Input: part model. Units: mm. Frame: model coordinates. Face numbers are marked on the shaded views. A direction names the side the tool comes from. Coordinates: 2 decimals unless noted, no trailing zeros. Order: outer loops, then holes, each group sorted by start corner. A loop starts at its lowest first (then second) coordinate and runs counter-clockwise, first axis right, second up. Notation, with made-up numbers: (85.5, -24) -> (105.5, -24) arc R25 ccw to (105.5, 1) -> close; hole circle Ø5 at (72, -36.75). An arc over 180 degrees is marked (long way). Use CSV: the item, a comma, the result in double quotes. Start each with the question number.
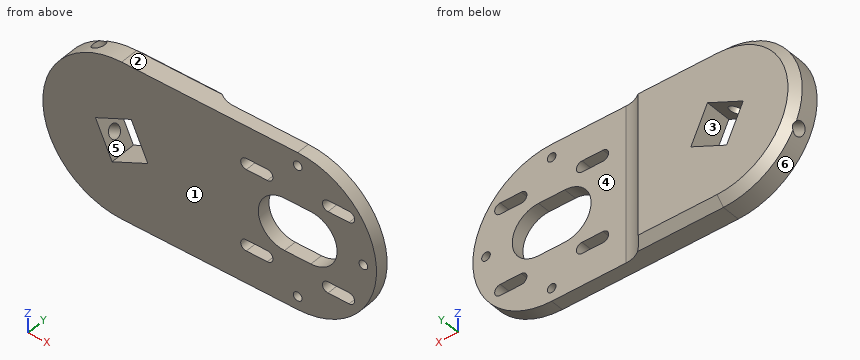
```python
from build123d import *

# Parameters (mm, degrees)
BOSS_EXTRUDE1_DEPTH = 5
CUT_EXTRUDE1_DEPTH  = 71.407741052
BOSS_EXTRUDE2_DEPTH = 5
FILLET1_R           = 10
CUT_EXTRUDE2_DEPTH  = 71.938353519
M4_TAPPED_HOLE1_D   = 3.3
SKETCH13_W          = 2.5
SKETCH13_H          = 32.367781463
SKETCH14_W          = 2.5
SKETCH14_H          = 32.367781463
CHAMFER1_SIZE       = 3


with BuildPart() as part:
    # Sketch1 → Boss-Extrude1 (new body)
    with BuildSketch(Plane(origin=(0, 0, 0), x_dir=(1, 0, 0), z_dir=(0, 1, 0))):
        with BuildLine():
            Line((-33.5, 30), (33.5, 30))
            ThreePointArc((33.5, 30), (63.5, 0), (33.5, -30))
            Line((33.5, -30), (-33.5, -30))
            ThreePointArc((-33.5, -30), (-63.5, 0), (-33.5, 30))
        make_face()
        with BuildLine():
            Line((28.5, 10), (38.5, 10))
            ThreePointArc((38.5, 10), (48.5, 0), (38.5, -10))
            Line((38.5, -10), (28.5, -10))
            ThreePointArc((28.5, -10), (18.5, 0), (28.5, 10))
        make_face(mode=Mode.SUBTRACT)
    extrude(amount=BOSS_EXTRUDE1_DEPTH)

    # Sketch2 → Cut-Extrude1 (cut, through all)
    with BuildSketch(Plane(origin=(0, 5, 0), x_dir=(1, 0, 0), z_dir=(0, 1, 0))):
        with BuildLine():
            Line((13.943650814, 17.686349186), (21.943650814, 17.686349186))
            ThreePointArc((21.943650814, 17.686349186), (24.073650814, 15.556349186), (21.943650814, 13.426349186))
            Line((21.943650814, 13.426349186), (13.943650814, 13.426349186))
            ThreePointArc((13.943650814, 13.426349186), (11.813650814, 15.556349186), (13.943650814, 17.686349186))
        make_face()
        with BuildLine():
            Line((53.056349186, 17.686349186), (45.056349186, 17.686349186))
            ThreePointArc((45.056349186, 17.686349186), (42.926349186, 15.556349186), (45.056349186, 13.426349186))
            Line((45.056349186, 13.426349186), (53.056349186, 13.426349186))
            ThreePointArc((53.056349186, 13.426349186), (55.186349186, 15.556349186), (53.056349186, 17.686349186))
        make_face()
        with BuildLine():
            Line((53.056349186, -17.686349186), (45.056349186, -17.686349186))
            ThreePointArc((45.056349186, -17.686349186), (42.926349186, -15.556349186), (45.056349186, -13.426349186))
            Line((45.056349186, -13.426349186), (53.056349186, -13.426349186))
            ThreePointArc((53.056349186, -13.426349186), (55.186349186, -15.556349186), (53.056349186, -17.686349186))
        make_face()
        with BuildLine():
            Line((13.943650814, -17.686349186), (21.943650814, -17.686349186))
            ThreePointArc((21.943650814, -17.686349186), (24.073650814, -15.556349186), (21.943650814, -13.426349186))
            Line((21.943650814, -13.426349186), (13.943650814, -13.426349186))
            ThreePointArc((13.943650814, -13.426349186), (11.813650814, -15.556349186), (13.943650814, -17.686349186))
        make_face()
    extrude(amount=-CUT_EXTRUDE1_DEPTH, mode=Mode.SUBTRACT)

    # Sketch8 → Boss-Extrude2 (add)
    with BuildSketch(Plane(origin=(0, 5, 0), x_dir=(1, 0, 0), z_dir=(0, 1, 0))):
        with BuildLine():
            ThreePointArc((-33.5, -30), (-12.286796564, -21.213203436), (-3.5, 0))
            ThreePointArc((-3.5, 0), (-12.286796564, 21.213203436), (-33.5, 30))
            ThreePointArc((-33.5, 30), (-63.5, 0), (-33.5, -30))
        make_face()
        with BuildLine():
            Line((-3.5, 0), (-3.5, 30))
            Line((-3.5, 30), (-33.5, 30))
            ThreePointArc((-33.5, 30), (-12.286796564, 21.213203436), (-3.5, 0))
        make_face()
        with BuildLine():
            Line((-3.5, -30), (-3.5, 0))
            ThreePointArc((-3.5, 0), (-12.286796564, -21.213203436), (-33.5, -30))
            Line((-33.5, -30), (-3.5, -30))
        make_face()
    extrude(amount=BOSS_EXTRUDE2_DEPTH)

    # Fillet1
    # the kernel refuses this fillet: 10 mm, written as the material it adds along each edge
    with BuildSketch(Plane(origin=(-3.5, 5, -30), x_dir=(0, 1, 0), z_dir=(0, 0, 1))) as fillet1_piece_1:
        with BuildLine():
            CenterArc((10, -8.660254038), FILLET1_R, 120, 60)
            Line((0, -8.660254038), (-0.2, -8.660254038))
            Line((-0.2, -8.660254038), (-0.2, 0))
            Line((-0.2, 0), (0, 0.2))
            ThreePointArc((0, 0.2), (2.5, 0.2), (4.9, 0.173205081))
            Line((4.9, 0.173205081), (5, 0))
        make_face()
    extrude(amount=60)

    # Sketch9 → Cut-Extrude2 (cut, through all)
    with BuildSketch(Plane(origin=(0, 10, 0), x_dir=(1, 0, 0), z_dir=(0, 1, 0))):
        Polygon((-43.466945366, -3.62767144), (-37.12767144, 9.966945366), (-23.533054634, 3.62767144), (-29.87232856, -9.966945366), align=None)
    extrude(amount=-CUT_EXTRUDE2_DEPTH, mode=Mode.SUBTRACT)

    # M4 Tapped Hole1 (through all)
    with Locations(Plane(origin=(0, 5, 0), x_dir=(1, 0, 0), z_dir=(0, 1, 0))):
        with Locations((33.5, 25), (33.5, -25), (58.5, 0)):
            Hole(M4_TAPPED_HOLE1_D / 2)

    # Sketch13 → M6 Tapped Hole1 (revolve, cut)
    with BuildSketch(Plane(origin=(-40.297308403, 5, -3.169636963), x_dir=(0.4226182617407039, 0, -0.9063077870366479), z_dir=(0, 1, 0))):
        with Locations((1.25, 16.183890732)):
            Rectangle(SKETCH13_W, SKETCH13_H)
    revolve(axis=Axis((-34.542253955, 5, -0.486011001), (-0.9063077870366478, 0, -0.4226182617407039)), mode=Mode.SUBTRACT)

    # Sketch14 → M6 Tapped Hole2 (revolve, cut)
    with BuildSketch(Plane(origin=(-36.669636963, 5, 6.797308403), x_dir=(-0.9063077870366478, 0, -0.42261826174070416), z_dir=(0, 1, 0))):
        with Locations((1.25, 16.183890732)):
            Rectangle(SKETCH14_W, SKETCH14_H)
    revolve(axis=Axis((-33.986011001, 5, 1.042253955), (-0.4226182617407042, 0, 0.9063077870366477)), mode=Mode.SUBTRACT)

    # Chamfer1
    # the kernel refuses this chamfer: 3 mm, written as the material it takes off along each edge
    with BuildSketch(Plane(origin=(-33.5, 10, 30), x_dir=(0, 0.02749587661058619, -0.9996219169112968), z_dir=(1, 0, 0)), Plane(origin=(4.215048964, 10, -30), x_dir=(0, 0.02749587661058619, 0.9996219169112968), z_dir=(-1, 0, 0))) as chamfer1_piece_1:
        Polygon((CHAMFER1_SIZE * 0.999621916911, -CHAMFER1_SIZE * 0.0274958766106), (-CHAMFER1_SIZE * 0.0274958766106, -CHAMFER1_SIZE * 0.999621916911), (0, 0), align=None)
    extrude(amount=37.715048964, mode=Mode.SUBTRACT)
    with BuildSketch(Plane(origin=(-33.5, 10, 0), x_dir=(0, 0, 1), z_dir=(1, 0, 0))) as chamfer1_piece_2:
        Polygon((30 - CHAMFER1_SIZE, 0), (30, CHAMFER1_SIZE), (30, 0), align=None)
    revolve(axis=Axis((-33.5, 10, 0), (0, -1, 0)), revolution_arc=180, mode=Mode.SUBTRACT)


solid = part.part
```
1. Access query for the marked faces 4, 5 and 6. Directions: +Z, -Z, +X, -X, +Y, -Y. A direction counts if a zero-diameter tool reaches every point of the face in a straight line with its end or side. Return the directions, or none.
2. Section C-C on x = 1. Return loops of the section in (y, z).
3. Section A-A on x = -32. Return loops of the section in (y, z), then the cut area to 3 significant figures.
4. Section B-B on x = 58.5. Return loops of the section in (y, z), then the cut area to 3 significant figures.
5. Pull-direction query (Z, two-part tool) for the marked faces 1, 2 and 3; classes: released by +Z, released by -Z, zero draft, split by the parting line, or undercut.
6. Contact query for flat-ended pins moving along their axis: P1, Ø5, axis at x = 41.5, z = -16, coming from the +Y side; P2, Ø2.5, axis at x = 49, y = 3.5, coming from the +Z side; P3, Ø1, axis at y = 5.5, z = -11.5, coming from the -X side; P4, Ø5.5, axis at x = 33.5, z = 25, coming from the -Y side. Output: stop coordinate, or through.
7. Material intervals for line 1 along Z through (x, y) = (33.5, 2.3); line 2 along X through (y, z) = (2.95, 25); line 3 along X through (y, z) = (4, -2), sorted ascending.
Values follow:
1,face 4,"+Z, -Z, +X, +Y"
1,face 5,"+Y, -Y"
1,face 6,"-X, +Y, -Y"
2,outline,"(0, -30) -> (5.91, -30) -> (5.91, 30) -> (0, 30) -> close"
3,outline,"(0, -30) -> (7, -30) -> (10, -27) -> (10, -7.58) -> (0, -7.58) -> close; (0, 8.97) -> (10, 8.97) -> (10, 27) -> (7, 30) -> (0, 30) -> close"
3,area,"425 mm2"
4,outline,"(0, -16.58) -> (5, -16.58) -> (5, -1.65) -> (0, -1.65) -> close; (0, 1.65) -> (5, 1.65) -> (5, 16.58) -> (0, 16.58) -> close"
4,area,"149 mm2"
5,face 1,"zero draft"
5,face 2,"released by +Z"
5,face 3,"undercut"
6,P1,"stops at y = 5"
6,P2,"stops at z = 26.4"
6,P3,"stops at x = -53.47"
6,P4,"stops at y = 0"
7,line 1,"z = -30 to -26.65, -23.35 to -10, 10 to 23.35, 26.65 to 30"
7,line 2,"x = -50.08 to -46.74, -43.58 to 31.85, 35.15 to 50.08"
7,line 3,"x = -63.43 to -43.21, -24.29 to 18.7, 48.3 to 63.43"
